Job drawing, mm, ordinate dimensions from the low corner. One solid piece. A direction names the side the tool comes from. Give positions to 0.01 mm unless a question says otherwise; leave off trailing zeros. Write each loop counter-clockwise with the first axis right and the second up, starting at its lowest first coordinate (ties: lowest second). Pieces come first, ordered by that corner, then holes. Notation, with made-up numbers: M 87,65 L 111,65 A19 cw 111,69 Z; hole C -37,-11 d3. An arc over 180 degrees is marked long. Answer as CSV lines item,"result". Start each with the question number.
Item 1: Wall check: L1, parallel to X at y = 43, z = 7; L2, parallel to Y at x = 96.5, z = 23; L3, parallel to Z at x = 94, y = 6.5. Give the ranges that are in metal, low to high. Write a range as from..to.
Item 2: Band-saw the part on A-A, the plane z = 9.5. List the corners of the cut face in (x, y).
Item 3: Pin check, flat tips, straight feed: pin 1 (5 mm diameter, centred on x = 98.425, y = 47.625, fed in from -Z); pin 2 (1.8 mm diameter, centred on x = 99, z = 1, fed in from +Y); pin 3 (4 mm diameter, centred on y = 4, z = 21.5, fed in from -X). Stop position of each tip, or through.
Item 4: 3-axis set-ups, long thin cutter, end or side, ignore diameter. For the marked faces 1, 2 and 3: which of +Z, -Z, +X, -X, +Y, -Y reach the whole face in a straight line?
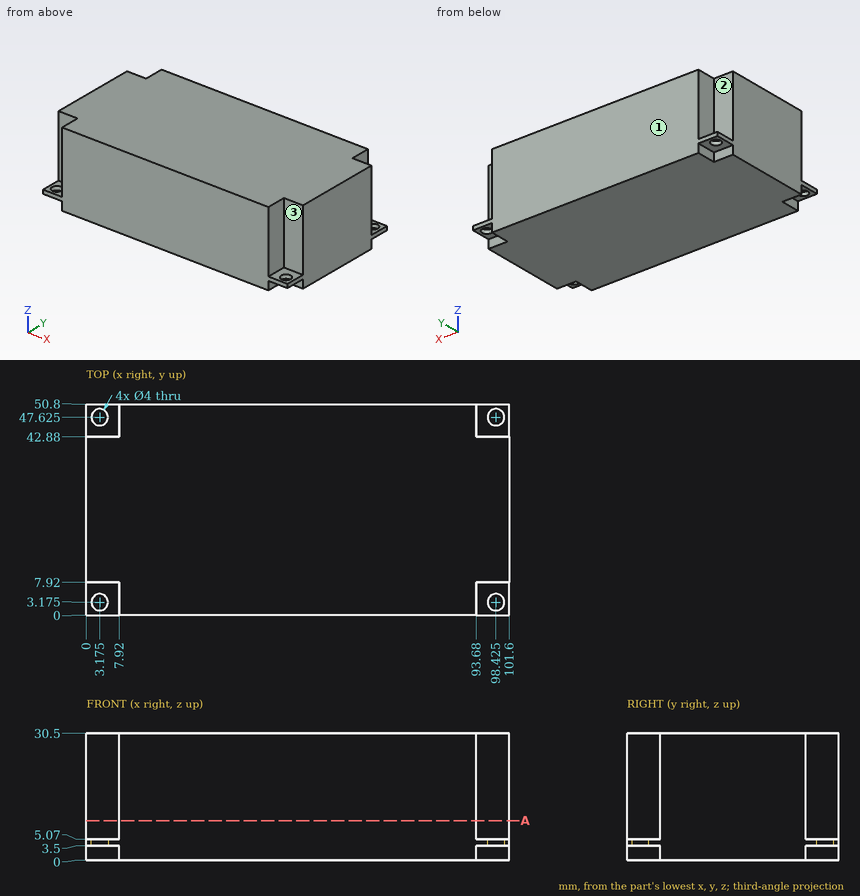
Output:
1,L1,"7.92..93.68"
1,L2,"7.92..42.88"
1,L3,"3.5..5.07"
2,outline,"M 0,7.92 L 7.92,7.92 L 7.92,0 L 93.68,0 L 93.68,7.92 L 101.6,7.92 L 101.6,42.88 L 93.68,42.88 L 93.68,50.8 L 7.92,50.8 L 7.92,42.88 L 0,42.88 Z"
3,pin 1,"z = 3.5"
3,pin 2,"y = 42.88"
3,pin 3,"x = 7.92"
4,face 1,"+Z, -Z, +X, -X, +Y"
4,face 2,"+Z, -X, +Y"
4,face 3,"+Z, +X, -Y"
